```python
from build123d import *

# Parameters (mm, degrees)
SKETCH1_R           = 1.651
SKETCH1_R_2         = 1.524
BOSS_EXTRUDE1_DEPTH = 6.35


with BuildPart() as part:
    # Sketch1 → Boss-Extrude1 (new body)
    with BuildSketch(Plane(origin=(0, 0, 0), x_dir=(1, 0, 0), z_dir=(0, 1, 0))):
        with BuildLine():
            Line((33.776652136, 18.187342636), (4.627239322, 18.187342636))
            Line((4.627239322, 18.187342636), (4.627239322, 33.034266248))
            Line((4.627239322, 33.034266248), (33.776652136, 33.034266248))
            Line((33.776652136, 33.034266248), (52.191652136, 33.034266248))
            Line((52.191652136, 33.034266248), (52.191652136, 57.360804442))
            Line((52.191652136, 57.360804442), (85.968304273, 57.360804442))
            Line((85.968304273, 57.360804442), (85.968304273, 76.214266248))
            Line((85.968304273, 76.214266248), (85.968304273, 79.389266248))
            Line((85.968304273, 79.389266248), (78.348304273, 79.389266248))
            Line((78.348304273, 79.389266248), (78.348304273, 76.214266248))
            Line((78.348304273, 76.214266248), (7.62, 76.214266248))
            Line((7.62, 76.214266248), (7.62, 79.389266248))
            Line((7.62, 79.389266248), (0, 79.389266248))
            Line((0, 79.389266248), (0, 76.214266248))
            Line((0, 76.214266248), (-12.371874213, 76.214266248))
            ThreePointArc((-12.371874213, 76.214266248), (-24.373410945, 58.595023332), (-30.932760678, 38.310804442))
            Line((-30.932760678, 38.310804442), (-15.692760678, 38.310804442))
            Line((-15.692760678, 38.310804442), (-15.692760678, 12.910804442))
            Line((-15.692760678, 12.910804442), (-30.932760678, 12.910804442))
            ThreePointArc((-30.932760678, 12.910804442), (-24.373410945, -7.373414447), (-12.371874213, -24.992657364))
            Line((-12.371874213, -24.992657364), (0, -24.992657364))
            Line((0, -24.992657364), (0, -28.167657364))
            Line((0, -28.167657364), (7.62, -28.167657364))
            Line((7.62, -28.167657364), (7.62, -24.992657364))
            Line((7.62, -24.992657364), (78.348304273, -24.992657364))
            Line((78.348304273, -24.992657364), (78.348304273, -28.167657364))
            Line((78.348304273, -28.167657364), (85.968304273, -28.167657364))
            Line((85.968304273, -28.167657364), (85.968304273, -24.992657364))
            Line((85.968304273, -24.992657364), (85.968304273, -6.139195558))
            Line((85.968304273, -6.139195558), (52.191652136, -6.139195558))
            Line((52.191652136, -6.139195558), (52.191652136, 18.187342636))
            Line((52.191652136, 18.187342636), (33.776652136, 18.187342636))
        make_face()
        with Locations(Location((3.357239322, -23.087657364, 0), (0, 0, 270))):
            Circle(SKETCH1_R, mode=Mode.SUBTRACT)
        with Locations(Location((82.611064951, -23.087657364, 0), (0, 0, 270))):
            Circle(SKETCH1_R, mode=Mode.SUBTRACT)
        with Locations(Location((42.984152136, -12.292657364, 0), (0, 0, 270))):
            Circle(SKETCH1_R_2, mode=Mode.SUBTRACT)
        with Locations(Location((42.984152136, -18.642657364, 0), (0, 0, 270))):
            Circle(SKETCH1_R_2, mode=Mode.SUBTRACT)
        with Locations(Location((42.984152136, -5.942657364, 0), (0, 0, 270))):
            Circle(SKETCH1_R_2, mode=Mode.SUBTRACT)
        with Locations(Location((42.984152136, 0.407342636, 0), (0, 0, 270))):
            Circle(SKETCH1_R_2, mode=Mode.SUBTRACT)
        with Locations(Location((42.984152136, 6.757342636, 0), (0, 0, 270))):
            Circle(SKETCH1_R_2, mode=Mode.SUBTRACT)
        with Locations(Location((42.984152136, 13.107342636, 0), (0, 0, 270))):
            Circle(SKETCH1_R_2, mode=Mode.SUBTRACT)
        with Locations(Location((42.984152136, 38.114266248, 0), (0, 0, 90))):
            Circle(SKETCH1_R_2, mode=Mode.SUBTRACT)
        with Locations(Location((82.611064951, 74.309266248, 0), (0, 0, 90))):
            Circle(SKETCH1_R, mode=Mode.SUBTRACT)
        with Locations(Location((3.357239322, 74.309266248, 0), (0, 0, 90))):
            Circle(SKETCH1_R, mode=Mode.SUBTRACT)
        with Locations(Location((-15.692760678, 59.900804442, 0), (0, 0, 270))):
            Circle(SKETCH1_R, mode=Mode.SUBTRACT)
        with Locations(Location((-15.692760678, -8.679195558, 0), (0, 0, 270))):
            Circle(SKETCH1_R, mode=Mode.SUBTRACT)
        with Locations(Location((42.984152136, 44.464266248, 0), (0, 0, 90))):
            Circle(SKETCH1_R_2, mode=Mode.SUBTRACT)
        with Locations(Location((42.984152136, 50.814266248, 0), (0, 0, 90))):
            Circle(SKETCH1_R_2, mode=Mode.SUBTRACT)
        with Locations(Location((42.984152136, 57.164266248, 0), (0, 0, 90))):
            Circle(SKETCH1_R_2, mode=Mode.SUBTRACT)
        with Locations(Location((42.984152136, 63.514266248, 0), (0, 0, 90))):
            Circle(SKETCH1_R_2, mode=Mode.SUBTRACT)
        with Locations(Location((42.984152136, 69.864266248, 0), (0, 0, 90))):
            Circle(SKETCH1_R_2, mode=Mode.SUBTRACT)
    extrude(amount=BOSS_EXTRUDE1_DEPTH)


solid = part.part
```
Geometry: final body of the model. Coordinates: model frame, mm. A direction names the side the tool comes from. Round coordinates to 2 decimals unless told otherwise and drop trailing zeros. Write each loop counter-clockwise with the first axis right and the second up, starting at its lowest first coordinate (ties: lowest second). Pieces come first, ordered by that corner, then holes. Notation, with made-up numbers: M -9,6 L 47,6 A36 cw 47,43 Z; hole C 36,-4.75 d6. An arc over 180 degrees is marked long. Answer in a Markdown table with one row per item. Add a question column.
(1) Ray query, L1, parallel to Z at x = 71, y = 2.5; L2, parallel to Z at x = 15, y = 5; L3, parallel to Z at x = -16, y = 2. Return the intervals inside material, ascending.
(2) Draft query along Z for faces 1 (the face through (43, 3, -76.214)), 2 (the face through (43.57, 3.13, -58.57)), 3 (the face through (52.192, 3, -45)), 4 (the face through (27, 0, -38)). Return one class per face: pulls with the +Z half, pulls with the -Z half, needs draft (parallel to the pull), parting line crosses it, or undercut.
(3) Contact query for flat-ended pins moving along their axis: pin 1 (2.5 mm diameter, centred on y = 2, z = -77.5, fed in from -X); pin 2 (1 mm diameter, centred on y = 3, z = -8.5, fed in from +X); pin 3 (1.9 mm diameter, centred on x = -9, y = 2.5, fed in from -Z). Output: stop coordinate, or through.
(4) Reachability of faces 5 (the face through (-23, 3, -38.311)), 6 (the face through (-16.325, 3.131, 10.204)), 7 (the face through (78.348, 3, 27)), 8 (the face through (28, 3, -33.034)) from +Z, -Z, +X, -X, +Y, -Y: full face, straight path, thin tool, end or side. Return the list, or none.
(5) Cut plane D-D, the plane x = -4. Return the cut outline in (y, z).
(6) Cut plane A-A, the plane x = 68. Return the cut outline in (y, z).
(7) Cut plane B-B, the plane x = 50. Return the cut outline in (y, z), then the cut area to 3 significant figures.
(8) Cut plane C-C, the plane z = -34.5. Return the cut outline in (x, y), then the cut area to 3 significant figures.
Established:
| question | item | result |
|---|---|---|
| 1 | L1 | -76.21 to -57.36, 6.14 to 24.99 |
| 1 | L2 | -76.21 to -33.03, -18.19 to 24.99 |
| 1 | L3 | -71.93 to -61.52, -58.28 to -38.31, -12.91 to 7.06, 10.3 to 20.71 |
| 2 | face 1 | pulls with the -Z half |
| 2 | face 2 | undercut |
| 2 | face 3 | undercut |
| 2 | face 4 | needs draft |
| 3 | pin 1 | x = 0 |
| 3 | pin 2 | x = 52.19 |
| 3 | pin 3 | z = -76.21 |
| 4 | face 5 | -X, +Y, -Y |
| 4 | face 6 | +Y, -Y |
| 4 | face 7 | +Z, +Y, -Y |
| 4 | face 8 | +X, +Y, -Y |
| 5 | outline | M 0,-76.21 L 6.35,-76.21 L 6.35,24.99 L 0,24.99 Z |
| 6 | outline | M 0,-76.21 L 6.35,-76.21 L 6.35,-57.36 L 0,-57.36 Z; M 0,6.14 L 6.35,6.14 L 6.35,24.99 L 0,24.99 Z |
| 7 | outline | M 0,-76.21 L 6.35,-76.21 L 6.35,-33.03 L 0,-33.03 Z; M 0,-18.19 L 6.35,-18.19 L 6.35,24.99 L 0,24.99 Z |
| 7 | area | 548 mm² |
| 8 | outline | M -15.69,0 L 52.19,0 L 52.19,6.35 L -15.69,6.35 Z |
| 8 | area | 431 mm² |
